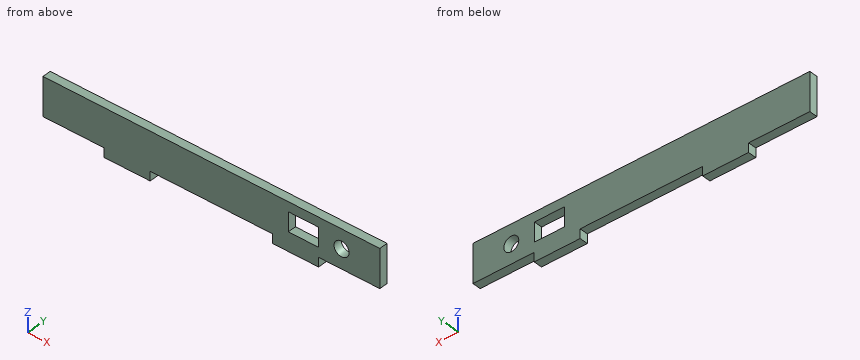
```python
from build123d import *

# Parameters (mm, degrees)
SKETCH1_W           = 30
SKETCH1_H           = 6
SKETCH1_W_2         = 220
SKETCH1_H_2         = 25
BOSS_EXTRUDE1_DEPTH = 5.5
SKETCH2_R           = 4.9
SKETCH2_W           = 19.6
SKETCH2_H           = 12.5
CUT_EXTRUDE1_DEPTH  = 112.680347421


with BuildPart() as part:
    # Sketch1 → Boss-Extrude1 (new body)
    with BuildSketch(Plane(origin=(0, 0, 0), x_dir=(1, 0, 0), z_dir=(0, 1, 0))):
        with Locations((-55, 15.5)):
            Rectangle(SKETCH1_W, SKETCH1_H)
        Rectangle(SKETCH1_W_2, SKETCH1_H_2)
        with Locations((55, 15.5)):
            Rectangle(SKETCH1_W, SKETCH1_H)
    extrude(amount=BOSS_EXTRUDE1_DEPTH)

    # Sketch2 → Cut-Extrude1 (cut, through all)
    with BuildSketch(Plane(origin=(0, 5.5, 0), x_dir=(1, 0, 0), z_dir=(0, 1, 0))):
        with Locations(Location((85, 0, 0), (0, 0, 270))):
            Circle(SKETCH2_R)
        with Locations((60, 0)):
            Rectangle(SKETCH2_W, SKETCH2_H)
    extrude(amount=-CUT_EXTRUDE1_DEPTH, mode=Mode.SUBTRACT)


solid = part.part
```
Input: part model. Units: mm. Frame: model coordinates. Give positions to 0.01 mm unless a question says otherwise; leave off trailing zeros. Write each loop counter-clockwise with the first axis right and the second up, starting at its lowest first coordinate (ties: lowest second). Pieces come first, ordered by that corner, then holes. Notation, with made-up numbers: (32.25, 11) - (36.25, 11) arc R30 ccw to (36.25, 33) - close; hole circle Ø10 at (73.25, -26). An arc over 180 degrees is marked (long way). Write item = value, one per line. Start each with the question number.
1. First-contact query: pin 1 Ø1.6 at (x, y) = (-97.5, 3.5) entering from -Z; pin 2 Ø1.6 at (y, z) = (2.5, -15.5) entering from +X. Flat tips, straight axial feed; report the tip coordinate or a pass-through.
2. Section query B-B, the plane z = 0. Output: boundary loops of the cut face in (x, y).
3. Ray query, L1, parallel to X at y = 1.7, z = 0; L2, parallel to X at y = 1.6, z = -17; L3, parallel to X at y = 0.55, z = 5. Return the intervals inside material, ascending.
4. Section query D-D, the plane x = -14.5. Output: boundary loops of the cut face in (y, z), then the cut area to 4 significant figures.
5. Section query C-C, the plane y = 4. Output: boundary loops of the cut face in (x, z), then the cut area to 3 significant figures.
6. Section query A-A, the plane x = 85. Output: boundary loops of the cut face in (y, z).
Check sheet entries:
q1.pin_1 = -12.5
q1.pin_2 = 70
q2.outline = (-110, 0) - (50.2, 0) - (50.2, 5.5) - (-110, 5.5) - close; (69.8, 0) - (80.1, 0) - (80.1, 5.5) - (69.8, 5.5) - close; (89.9, 0) - (110, 0) - (110, 5.5) - (89.9, 5.5) - close
q3.L1 = -110 to 50.2, 69.8 to 80.1, 89.9 to 110
q3.L2 = -70 to -40, 40 to 70
q3.L3 = -110 to 50.2, 69.8 to 110
q4.outline = (0, -12.5) - (5.5, -12.5) - (5.5, 12.5) - (0, 12.5) - close
q4.area = 137.5 mm2
q5.outline = (-110, -12.5) - (-70, -12.5) - (-70, -18.5) - (-40, -18.5) - (-40, -12.5) - (40, -12.5) - (40, -18.5) - (70, -18.5) - (70, -12.5) - (110, -12.5) - (110, 12.5) - (-110, 12.5) - close; hole (50.2, -6.25) - (69.8, -6.25) - (69.8, 6.25) - (50.2, 6.25) - close; hole circle Ø9.8 at (85, 0)
q5.area = 5,540 mm2
q6.outline = (0, -12.5) - (5.5, -12.5) - (5.5, -4.9) - (0, -4.9) - close; (0, 4.9) - (5.5, 4.9) - (5.5, 12.5) - (0, 12.5) - close
